from build123d import *
from OCP.BRepFilletAPI import BRepFilletAPI_MakeChamfer

# Parameters (mm, degrees)
BOSS_EXTRUDE1_DEPTH = 4.5
CHAMFER1_SIZE       = 2
CHAMFER1_SIZE2      = 5.494954839


with BuildPart() as part:
    # Sketch1 → Boss-Extrude1 (new body)
    with BuildSketch(Plane.XY):
        Polygon((-42.5, -25.6), (-42.5, -30.6), (42.5, -30.6), (42.5, 30.6), (-42.5, 30.6), (-42.5, 25.6), (37.5, 25.6), (37.5, -25.6), align=None)
    extrude(amount=BOSS_EXTRUDE1_DEPTH)

    # Chamfer1: one chamfer whose edges measure the first distance from different faces: ONE call of the kernel's chamfer builder (chamfer() names one face for all edges)
    chamfer1_edges_1 = [part.edges().sort_by_distance(p)[0] for p in [
        (42.5, -30.6, 2.25),
    ]]
    chamfer1_side_1 = [part.faces().sort_by_distance(p)[0] for p in [
        (0, -30.6, 2.25),
    ]]
    chamfer1_edges_2 = [part.edges().sort_by_distance(p)[0] for p in [
        (42.5, 30.6, 2.25),
    ]]
    chamfer1_side_2 = [part.faces().sort_by_distance(p)[0] for p in [
        (0, 30.6, 2.25),
    ]]
    chamfer1 = BRepFilletAPI_MakeChamfer(part.part.solid().wrapped)
    for e in chamfer1_edges_1:
        chamfer1.Add(CHAMFER1_SIZE, CHAMFER1_SIZE2, e.wrapped, chamfer1_side_1[0].wrapped)  # the first distance lies on this face
    for e in chamfer1_edges_2:
        chamfer1.Add(CHAMFER1_SIZE, CHAMFER1_SIZE2, e.wrapped, chamfer1_side_2[0].wrapped)  # the first distance lies on this face
    add(Compound.cast(chamfer1.Shape()), mode=Mode.REPLACE)


solid = part.part
Verification items for the finished model (mm, model axes). A direction names the side the tool comes from. Coordinates: 2 decimals unless noted, no trailing zeros. Order: outer loops, then holes, each group sorted by start corner. A loop starts at its lowest first (then second) coordinate and runs counter-clockwise, first axis right, second up.
1. Release check for a two-part mould opening along Y. For faces 1 (the face through (9, -27, 0)), 2 (the face through (-3, 25.6, 2)), 3 (the face through (41.514, 27.814, 2.218)) record: +Y half, -Y half, draft (parallel to the pull), parting line (faces both ways), or undercut.
Results found:
face 1: draft
face 2: undercut
face 3: +Y half
2. Scan lines: line 1 (Y direction, x = 13, z = 0.25); line 2 (X direction, y = -18.5, z = 3.25); line 3 (X direction, y = 25.5, z = 3.2). Record each from-to range of solid material in increasing order.
Results found:
line 1: y = -30.6 to -25.6, 25.6 to 30.6
line 2: x = 37.5 to 42.5
line 3: x = 37.5 to 42.36
3. Sectioned sample at B-B, the plane z = 1.95. Record the cut outline in (x, y), and give its area (3 significant figures).
Results found:
outline: (-42.5, -30.6) - (40.5, -30.6) - (42.5, -25.11) - (42.5, 25.11) - (40.5, 30.6) - (-42.5, 30.6) - (-42.5, 25.6) - (37.5, 25.6) - (37.5, -25.6) - (-42.5, -25.6) - close
area: 1,100 mm2
4. Set-up check for faces 4 (the face through (9, -27, 4.5)), 5 (the face through (-2, -25.6, 2)): record each of +Z, -Z, +X, -X, +Y, -Y from which the full face is reachable in a straight line by a thin tool's end or side.
Results found:
face 4: +Z, +X, -X, +Y, -Y
face 5: +Z, -Z, -X
5. Sectioned sample at C-C, the plane y = -22. Record the cut outline in (x, z), and give its area (3 significant figures).
Results found:
outline: (37.5, 0) - (42.5, 0) - (42.5, 4.5) - (37.5, 4.5) - close
area: 22.5 mm2
6. Sectioned sample at A-A, the plane x = 13.5. Record the cut outline in (y, z), and give its area (3 significant figures).
Results found:
outline: (-30.6, 0) - (-25.6, 0) - (-25.6, 4.5) - (-30.6, 4.5) - close; (25.6, 0) - (30.6, 0) - (30.6, 4.5) - (25.6, 4.5) - close
area: 45.0 mm2
